Autodesk Inventor part; units mm, degrees
ref_plane "YZ Plane" through (0, 0, 0) normal (1, 0, 0) x (0, 1, 0)
ref_plane "XZ Plane" through (0, 0, 0) normal (0, 1, 0) x (-1, 0, 0)
ref_plane "XY Plane" through (0, 0, 0) normal (0, 0, 1) x (1, 0, 0)
sketch "スケッチ1" plane through (0, 0, 0) normal (0, 1, 0) x (-1, 0, 0)
  arc A0 (72.9254, -25.3463) -> (139.4294, -19.0858) centre (64.9013, 416.2515) ccw
  arc A1 (54.1052, -25.1311) -> (72.9254, -25.3463) centre (67.1484, 292.5868) ccw
  arc A2 (19.6951, -19.0145) -> (54.1052, -25.1311) centre (59.4352, 104.7024) ccw
  arc A3 (-0.0609, -9.311) -> (19.6951, -19.0145) centre (42.8692, 53.13) ccw
  arc A4 (-5.5029, -4.0266) -> (-0.0609, -9.311) centre (12.76, 9.3368) ccw
  arc A5 (-2.9938, 3.6874) -> (-5.5029, -4.0266) centre (-1.4678, -1.074) ccw
  arc A6 (5.1717, 4.7562) -> (-2.9938, 3.6874) centre (4.0256, -18.2153) ccw
  arc A7 (36.109, -0.9508) -> (5.1717, 4.7562) centre (-0.7578, -114.096) ccw
  arc A8 (36.109, -0.9508) -> (38.0145, -1.5673) centre (185.125, 456.3841) ccw
  arc A9 (38.0145, -1.5673) -> (139.3334, -17.8944) centre (142.307, 323.0926) ccw
  arc A10 (139.4294, -19.0858) -> (139.3334, -17.8944) centre (139.3282, -18.4944) ccw
  circle A11 centre (6.8478, -1.4519) radius 3
  circle A12 centre (92.934, -19.7045) radius 3
  point P0 (0, 0)
extrude "押し出し1" add sketch "スケッチ1" along normal mid plane 186 contours A1 A2 A3 A4 A5 A6 A7 A8 A9 A10 A0 | A11 | A12
shell "シェル1" thickness 1 outward yes removed faces 2 at (-47.7634, 93, -11.4021) at (-47.7634, -93, -11.4021)
properties part number "GFRP_sub"
Can you work these out from the model? Positions are in its coordinate system, mm. A direction names the side the tool comes from. Give positions to 0.01 mm unless a question says otherwise; leave off trailing zeros. Loops run counter-clockwise (first coordinate to the right, second up) from the corner with the lowest first, then second, coordinate; pieces in that order, holes last. Notation, with made-up numbers: (-28, 25) -> (14, 25) arc R11 ccw to (14, 37) -> close; hole circle Ø2 at (-32.5, 76.5). An arc over 180 degrees is marked (long way). Return JSON: item names as keys, results as strings.
Q1. For pin 1 Ø1 at (y, z) = (42.5, -4) entering from +X; pin 2 Ø5 at (x, y) = (-120.5, -50.5) entering from +Z; pin 3 Ø3 at (y, z) = (40.5, -3) entering from +X, each with a flat end and sliding along its axis, tell me the tip position at first contact or that it passes through.
Checks:
{"pin 1": "stops at x = 6.96", "pin 2": "stops at z = -16.04", "pin 3": "stops at x = 7.45"}
Q2. We'd pull the mould along Z, two halves only. Please class faces 3 (the face through (-8.88, 1.3, -15.71)), 4 (the face through (-63.382, 1.302, -25.376)), 5 (the face through (-9.324, 1.302, -14.816)), 6 (the face through (-66, -93, -9)): released by +Z, released by -Z, zero draft, split by the parting line, or undercut.
Checks:
{"face 3": "released by -Z", "face 4": "undercut", "face 5": "undercut", "face 6": "zero draft"}
Q3. I want a section at A-A, the plane x = -129. List the corners of the cut face in (y, z) for me.
Checks:
{"outline": "(-93, -21.75) -> (93, -21.75) -> (93, -20.74) -> (-93, -20.74) -> close; (-93, -17.65) -> (93, -17.65) -> (93, -16.65) -> (-93, -16.65) -> close"}
Q4. I want a section at C-C, the plane x = -17. List the corners of the cut face in (y, z) for me.
Checks:
{"outline": "(-93, -19.16) -> (93, -19.16) -> (93, -18.09) -> (-93, -18.09) -> close; (-93, 3.57) -> (93, 3.57) -> (93, 4.58) -> (-93, 4.58) -> close"}
Q5. I want a section at B-B, the plane y = 29. List the corners of the cut face in (x, z) for me, then the cut area to 3 significant figures.
Checks:
{"outline": "(-139.6, -20.07) arc R442.67 ccw to (-72.94, -26.35) arc R319.06 ccw to (-54.06, -26.13) arc R130.94 ccw to (-19.39, -19.97) arc R76.77 ccw to (0.63, -10.14) arc R23.63 ccw to (6.31, -4.62) arc R6 ccw to (3.3, 4.64) arc R24 ccw to (-5.22, 5.75) arc R120 ccw to (-36.42, 0) arc R481.19 cw to (-38.32, -0.62) arc R340 cw to (-139.34, -16.89) arc R1.6 ccw to start; hole (-139.43, -19.09) arc R441.67 ccw to (-72.93, -25.35) arc R318.06 ccw to (-54.11, -25.13) arc R129.94 ccw to (-19.7, -19.01) arc R75.77 ccw to (0.06, -9.31) arc R22.63 ccw to (5.5, -4.03) arc R5 ccw to (2.99, 3.69) arc R23 ccw to (-5.17, 4.76) arc R119 ccw to (-36.11, -0.95) arc R482.19 cw to (-38.01, -1.57) arc R341 cw to (-139.33, -17.89) arc R0.6 ccw to start", "area": "310 mm2"}
Q6. On a 3-axis mill with a long thin cutter (end or side, diameter ignored), from which of +Z, -Z, +X, -X, +Y, -Y can I reach the whole of each face in a straight line? I mean faces 1 (the face through (-1.098, 1.302, 4.598)), 2 (the face through (-87.506, 1.302, -12.462)). Say none if no direction works.
Checks:
{"face 1": "+Y, -Y", "face 2": "+Z, -X, +Y, -Y"}
Q7. I need wall thicknesses on probe 1 along Z at (x, y) = (-92.5, 71.5); probe 2 along Z at (x, y) = (-75, -31). Which ranges of each line are inside material? Lowest first, please.
Checks:
{"probe 1": "z = -25.56 to -24.56, -14.25 to -13.24", "probe 2": "z = -26.3 to -25.3, -11.2 to -10.18"}
